```python
from build123d import *

# Parameters (mm, degrees)
SKETCH1_W           = 48.472676838
SKETCH1_H           = 40.157820008
BOSS_EXTRUDE1_DEPTH = 12.7
SKETCH3_W           = 40.64
SKETCH3_H           = 40.157820008
CUT_EXTRUDE2_DEPTH  = 6.35
FILLET7_R           = 3.81
SKETCH4_W           = 7.832676838
SKETCH4_H           = 40.157820008
CUT_EXTRUDE3_DEPTH  = 2.54
CUT_EXTRUDE4_DEPTH  = 129.54


with BuildPart() as part:
    # Sketch1 → Boss-Extrude1 (new body)
    with BuildSketch(Plane.XY):
        with Locations((5.884543073, 14.710946933)):
            Rectangle(SKETCH1_W, SKETCH1_H)
    extrude(amount=BOSS_EXTRUDE1_DEPTH)

    # Sketch3 → Cut-Extrude2 (cut)
    with BuildSketch(Plane.XY.offset(12.7)):
        with Locations((1.968204654, 14.710946933)):
            Rectangle(SKETCH3_W, SKETCH3_H)
    extrude(amount=-CUT_EXTRUDE2_DEPTH, mode=Mode.SUBTRACT)

    # Fillet7
    fillet7_edges = [part.edges().sort_by_distance(p)[0] for p in [
        (22.288204654, 14.710946933, 6.35),
    ]]
    fillet(fillet7_edges, radius=FILLET7_R)

    # Sketch4 → Cut-Extrude3 (cut)
    with BuildSketch(Plane.XY.offset(12.7)):
        with Locations((26.204543073, 14.710946933)):
            Rectangle(SKETCH4_W, SKETCH4_H)
    extrude(amount=-CUT_EXTRUDE3_DEPTH, mode=Mode.SUBTRACT)

    # Sketch5 → Cut-Extrude4 (cut)
    with BuildSketch(Plane(origin=(0, 34.789856937, 0), x_dir=(1, 0, 0), z_dir=(0, 1, 0))):
        Polygon((-18.351795346, 0), (-18.351795346, -6.35), (-2.210194986, 0), align=None)
    extrude(amount=-CUT_EXTRUDE4_DEPTH, mode=Mode.SUBTRACT)


solid = part.part
```
Could you check a few things on this model? Use its own coordinates, in mm. A direction names the side the tool comes from. Coordinates: 2 decimals unless noted, no trailing zeros. Order: outer loops, then holes, each group sorted by start corner. A loop starts at its lowest first (then second) coordinate and runs counter-clockwise, first axis right, second up. Notation, with made-up numbers: M -39.5,38.5 L -9.5,38.5 A21 ccw -9.5,44.5 Z; hole C 65,80.25 d5. An arc over 180 degrees is marked long. Use one line per item in the form item = value. Start each with the question number.
1. Suppose I cut it at C-C on z = 5.25. Write out the boundary of the cut face in (x, y), then the cut area to 3 significant figures.
2. Suppose I cut it at A-A on y = -3. Write out the boundary of the cut face in (x, z), then the cut area to 3 significant figures.
3. Please list where these lines run through material, in increasing order: line 1 (Z direction, x = -1, y = -2); line 2 (X direction, y = 18, z = 8.75); line 3 (Z direction, x = -8.5, y = 4).
4. On a 3-axis mill with a long thin cutter (end or side, diameter ignored), from which of +Z, -Z, +X, -X, +Y, -Y can I reach the whole of each face in a straight line? I mean faces 1 (the flat face through (11, -5.368, 4)), 2 (the flat face through (0, 15, 6.35)). Say none if no direction works.
5. Suppose I cut it at B-B on x = 0. Write out the boundary of the cut face in (y, z), then the cut area to 3 significant figures.
6. For pin 1 (6 mm diameter, centred on x = 9.5, y = 19, fed in from +Z); pin 2 (10 mm diameter, centred on x = 18.5, y = -0.5, fed in from -Z); pin 3 (8 mm diameter, centred on x = -8.5, y = 30, fed in from -Z), each with a flat end and sliding along its axis, tell me the tip position at first contact or that it passes through.
Geometry says:
q1.outline = M -15.56,-5.37 L 30.12,-5.37 L 30.12,34.79 L -15.56,34.79 Z
q1.area = 1,830 mm^2
q2.outline = M -18.35,6.35 L -2.21,0 L 30.12,0 L 30.12,10.16 L 22.29,10.16 A3.81 cw 18.48,6.35 Z
q2.area = 290 mm^2
q3.line_1 = 0 to 6.35
q3.line_2 = 22.02 to 30.12
q3.line_3 = 2.47 to 6.35
q4.face_1 = +Z, -Z, +X, -X, -Y
q4.face_2 = +Z, -X, +Y, -Y
q5.outline = M -5.37,0 L 34.79,0 L 34.79,6.35 L -5.37,6.35 Z
q5.area = 255 mm^2
q6.pin_1 = 6.35
q6.pin_2 = 0
q6.pin_3 = 0.9
